Verification items for the finished model (mm, model axes). A direction names the side the tool comes from. Round coordinates to 2 decimals unless told otherwise and drop trailing zeros. Write each loop counter-clockwise with the first axis right and the second up, starting at its lowest first coordinate (ties: lowest second). Pieces come first, ordered by that corner, then holes. Notation, with made-up numbers: (42, 41.25) - (92, 41.25) arc R5 cw to (92, 47.25) - close; hole circle Ø10 at (76, 68). An arc over 180 degrees is marked (long way). Answer as a JSON object with one key per item and string values. Group by question number.
1) Section check A-A (z = 3). Enter the section's corners in (x, y).
2) Go/stop test with flat-tipped pins: pin 1 Ø4 at (y, z) = (1, 39) entering from -X; pin 2 Ø4 at (x, z) = (3, -42) entering from -Y. Record where each tip stops, or that it passes through.
3) Thickness scan on line 1 (Z direction, x = -2.75, y = 0.25); line 2 (Y direction, x = 0, z = -54); line 3 (Y direction, x = -0.75, z = 36.5). Record the ranges inside material, lowest first.
4) Mould release check, pull along Z, two halves, no side actions. Record for faces 3 (the cylindrical face through (-0.401, -1.806, 0.984)), 4 (the flat face through (0, 0, 72.25)), 5 (the flat face through (0, 0, -72.25)): +Z half, -Z half, draft (parallel to the pull), parting line (faces both ways), or undercut.
5) Set-up check for faces 1 (the flat face through (-1, 2, -70.25)), 2 (the cylindrical face through (-3.695, -1.532, 71.091)): record each of +Z, -Z, +X, -X, +Y, -Y from which the full face is reachable in a straight line by a thin tool's end or side.
```python
from build123d import *

# Parameters (mm, degrees)
SKETCH1_R                = 1.85
BOSS_EXTRUDE1_DEPTH      = 70.25
SKETCH2_R                = 4
BOSS_EXTRUDE2_DEPTH      = 2
CHAMFER1_SIZE            = 0.5
FILLET2_R                = 0.25
FILLET3_R                = 0.125
CHAMFER1_OF_MIRROR2_SIZE = 0.5
FILLET2_OF_MIRROR2_R     = 0.25
FILLET3_OF_MIRROR2_R     = 0.125


with BuildPart() as part:
    # Sketch1 → Boss-Extrude1 (new body, symmetric)
    with BuildSketch(Plane.XY):
        Circle(SKETCH1_R)
    extrude(amount=BOSS_EXTRUDE1_DEPTH, both=True)

    # Sketch2 → Boss-Extrude2 (add)
    with BuildSketch(Plane(origin=(0, 0, -70.25), x_dir=(-1, 0, 0), z_dir=(0, 0, -1))):
        Circle(SKETCH2_R)
    boss_extrude2 = extrude(amount=BOSS_EXTRUDE2_DEPTH)

    # Chamfer1
    chamfer1_edges = [part.edges().sort_by_distance(p)[0] for p in [
        (4, 0, -72.25),
    ]]
    chamfer(chamfer1_edges, length=CHAMFER1_SIZE)

    # Fillet2
    fillet2_edges = [part.edges().sort_by_distance(p)[0] for p in [
        (4, 0, -70.25),
    ]]
    fillet(fillet2_edges, radius=FILLET2_R)

    # Fillet3
    fillet3_edges = [part.edges().sort_by_distance(p)[0] for p in [
        (4, 0, -71.75),
        (3.5, 0, -72.25),
    ]]
    fillet(fillet3_edges, radius=FILLET3_R)

    # Mirror2: Boss-Extrude2 across plane
    add(boss_extrude2.mirror(Plane.XY))

    # Chamfer1 of Mirror2
    chamfer1_of_mirror2_edges = [part.edges().sort_by_distance(p)[0] for p in [
        (4, 0, 72.25),
    ]]
    chamfer(chamfer1_of_mirror2_edges, length=CHAMFER1_OF_MIRROR2_SIZE)

    # Fillet2 of Mirror2
    fillet2_of_mirror2_edges = [part.edges().sort_by_distance(p)[0] for p in [
        (4, 0, 70.25),
    ]]
    fillet(fillet2_of_mirror2_edges, radius=FILLET2_OF_MIRROR2_R)

    # Fillet3 of Mirror2
    fillet3_of_mirror2_edges = [part.edges().sort_by_distance(p)[0] for p in [
        (4, 0, 71.75),
        (3.5, 0, 72.25),
    ]]
    fillet(fillet3_of_mirror2_edges, radius=FILLET3_OF_MIRROR2_R)


solid = part.part
```
Returned:
{
 "1": {"outline": "circle Ø3.7 at (0, 0)"},
 "2": {"pin 1": "x = -1.85", "pin 2": "y = -1.56"},
 "3": {"line 1": "-72.25 to -70.25, 70.25 to 72.25", "line 2": "-1.85 to 1.85", "line 3": "-1.69 to 1.69"},
 "4": {"face 3": "undercut", "face 4": "+Z half", "face 5": "-Z half"},
 "5": {"face 1": "none", "face 2": "+Z, -Z"}
}
